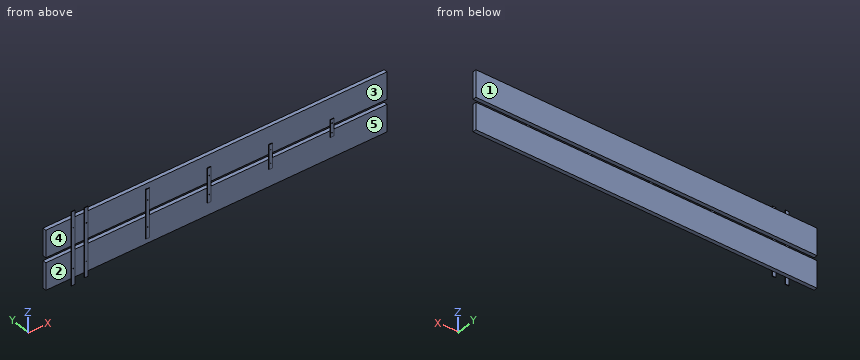
```python
from build123d import *

# Parameters (mm, degrees)
SKETCH2_W             = 19.05
SKETCH2_H             = 355.00056
SKETCH2_R             = 2
BOSS_EXTRUDE1_DEPTH   = 3.175
SKETCH2_H_2           = 251.02058
BOSS_EXTRUDE1_2_DEPTH = 3.175
SKETCH2_H_3           = 177.45456
BOSS_EXTRUDE1_3_DEPTH = 3.175
SKETCH2_H_4           = 125.44806
BOSS_EXTRUDE1_4_DEPTH = 3.175
SKETCH2_H_5           = 88.64092
BOSS_EXTRUDE1_5_DEPTH = 3.175
SKETCH2_H_6           = 376.10796
BOSS_EXTRUDE1_6_DEPTH = 3.175
SKETCH3_W             = 1788.19
SKETCH3_H             = 140
BOSS_EXTRUDE2_DEPTH   = 19


with BuildPart() as part:
    # Sketch2 → Boss-Extrude1 (new body)
    with BuildSketch(Plane(origin=(0, 0, 0), x_dir=(1, 0, 0), z_dir=(0, 1, 0))):
        with Locations((32.525, 177.50028)):
            Rectangle(SKETCH2_W, SKETCH2_H)
        with Locations((32.525, 79.875126)):
            Circle(SKETCH2_R, mode=Mode.SUBTRACT)
        with Locations((32.525, 275.125434)):
            Circle(SKETCH2_R, mode=Mode.SUBTRACT)
    extrude(amount=BOSS_EXTRUDE1_DEPTH)



with BuildPart() as body_2:
    # Sketch2 → Boss-Extrude1 2 (new body)
    with BuildSketch(Plane(origin=(0, 0, 0), x_dir=(1, 0, 0), z_dir=(0, 1, 0))):
        with Locations((354.525, 177.50028)):
            Rectangle(SKETCH2_W, SKETCH2_H_2)
        with Locations((354.525, 108.48022915)):
            Circle(SKETCH2_R, mode=Mode.SUBTRACT)
        with Locations((354.525, 246.52033085)):
            Circle(SKETCH2_R, mode=Mode.SUBTRACT)
    extrude(amount=BOSS_EXTRUDE1_2_DEPTH)


with BuildPart() as body_3:
    # Sketch2 → Boss-Extrude1 3 (new body)
    with BuildSketch(Plane(origin=(0, 0, 0), x_dir=(1, 0, 0), z_dir=(0, 1, 0))):
        with Locations((676.525, 177.50028)):
            Rectangle(SKETCH2_W, SKETCH2_H_3)
        with Locations((676.525, 128.708539125)):
            Circle(SKETCH2_R, mode=Mode.SUBTRACT)
        with Locations((676.525, 226.292020875)):
            Circle(SKETCH2_R, mode=Mode.SUBTRACT)
    extrude(amount=BOSS_EXTRUDE1_3_DEPTH)


with BuildPart() as body_4:
    # Sketch2 → Boss-Extrude1 4 (new body)
    with BuildSketch(Plane(origin=(0, 0, 0), x_dir=(1, 0, 0), z_dir=(0, 1, 0))):
        with Locations((998.525, 177.50028)):
            Rectangle(SKETCH2_W, SKETCH2_H_4)
        with Locations((998.525, 143.008361365)):
            Circle(SKETCH2_R, mode=Mode.SUBTRACT)
        with Locations((998.525, 211.992198635)):
            Circle(SKETCH2_R, mode=Mode.SUBTRACT)
    extrude(amount=BOSS_EXTRUDE1_4_DEPTH)


with BuildPart() as body_5:
    # Sketch2 → Boss-Extrude1 5 (new body)
    with BuildSketch(Plane(origin=(0, 0, 0), x_dir=(1, 0, 0), z_dir=(0, 1, 0))):
        with Locations((1320.525, 177.50028)):
            Rectangle(SKETCH2_W, SKETCH2_H_5)
        with Locations((1320.525, 153.11720963)):
            Circle(SKETCH2_R, mode=Mode.SUBTRACT)
        with Locations((1320.525, 201.88335037)):
            Circle(SKETCH2_R, mode=Mode.SUBTRACT)
    extrude(amount=BOSS_EXTRUDE1_5_DEPTH)


with BuildPart() as body_6:
    # Sketch2 → Boss-Extrude1 6 (new body)
    with BuildSketch(Plane(origin=(0, 0, 0), x_dir=(1, 0, 0), z_dir=(0, 1, 0))):
        with Locations((-36.475, 177.50028)):
            Rectangle(SKETCH2_W, SKETCH2_H_6)
        with Locations((-36.475, 74.070591)):
            Circle(SKETCH2_R, mode=Mode.SUBTRACT)
        with Locations((-36.475, 280.929969)):
            Circle(SKETCH2_R, mode=Mode.SUBTRACT)
    extrude(amount=BOSS_EXTRUDE1_6_DEPTH)


with BuildPart() as part_1:
    add(part.part)

    add(body_2.part)  # Boss-Extrude2 merges body 2

    add(body_3.part)  # Boss-Extrude2 merges body 3

    add(body_4.part)  # Boss-Extrude2 merges body 4

    add(body_5.part)  # Boss-Extrude2 merges body 5

    add(body_6.part)  # Boss-Extrude2 merges body 6
    # Sketch3 → Boss-Extrude2 (add)
    with BuildSketch(Plane(origin=(0, 3.175, 0), x_dir=(1, 0, 0), z_dir=(0, 1, 0))):
        with Locations((716.71, 260.20028)):
            Rectangle(SKETCH3_W, SKETCH3_H)
        with Locations((716.71, 94.80028)):
            Rectangle(SKETCH3_W, SKETCH3_H)
    extrude(amount=BOSS_EXTRUDE2_DEPTH)


solid = part_1.part
```
CAD build for the part. Positions are in the model's coordinates, mm. Face numbers are marked on the shaded views. A direction names the side the tool comes from. Round coordinates to 2 decimals unless told otherwise and drop trailing zeros. Write each loop counter-clockwise with the first axis right and the second up, starting at its lowest first coordinate (ties: lowest second). Pieces come first, ordered by that corner, then holes. Notation, with made-up numbers: M 40.25,65 L 81.25,65 A17 ccw 81.25,90 Z; hole C 5,-36 d1. An arc over 180 degrees is marked long. One line per question, with ' | ' between items.
1. Pin check, flat tips, straight feed: pin 1 Ø8 at (x, y) = (18, 15.5) entering from -Z; pin 2 Ø9.5 at (x, y) = (640.5, 12) entering from +Z; pin 3 Ø8 at (x, z) = (1306, -50.5) entering from -Y (3 decimals). Stop position of each tip, or through.
Working result:
pin 1: z = -330.2 | pin 2: z = -24.8 | pin 3: y = 3.175
2. Cut at B-B on x = 1354. Write the cut outline in (y, z) (3 decimals).
Working result:
outline: M 3.175,-330.2 L 22.175,-330.2 L 22.175,-190.2 L 3.175,-190.2 Z; M 3.175,-164.8 L 22.175,-164.8 L 22.175,-24.8 L 3.175,-24.8 Z
3. Which spindle directions (+Z, -Z, +X, -X, +Y, -Y) get a long thin tool onto all of the face, cutting with end or side? Do the marked faces 1 and 2. Say none if no direction does.
Working result:
face 1: +Z, -Z, +X, -X, +Y | face 2: +Z, -Z, -X, -Y
4. Mould opens along X. For the marked faces 3, 4 and 5 say: pulls with the +X half, pulls with the -X half, needs draft (parallel to the pull), parting line crosses it, or undercut.
Working result:
face 3: undercut | face 4: needs draft | face 5: undercut
5. Cut at A-A on y = 18.5. Write the cut outline in (x, z) (3 decimals), and give its area (3 significant figures).
Working result:
outline: M -177.385,-330.2 L 1610.805,-330.2 L 1610.805,-190.2 L -177.385,-190.2 Z; M -177.385,-164.8 L 1610.805,-164.8 L 1610.805,-24.8 L -177.385,-24.8 Z | area: 501,000 mm2
6. Probe L1, parallel to X at y = 1, z = -266; L2, parallel to Z at x = -5.5, y = 19.75; L3, parallel to Y at x = 631.5, z = -94 (3 decimals). List the from-to ranges inside material, lowest first. Write a range as from..to.
Working result:
L1: -46..-26.95, 23..42.05, 345..364.05, 667..686.05 | L2: -330.2..-190.2, -164.8..-24.8 | L3: 3.175..22.175
